The model under review builds one solid part; all positions refer to its coordinate system, in mm. A direction names the side the tool comes from. Give positions to 0.01 mm unless a question says otherwise; leave off trailing zeros. Order: outer loops, then holes, each group sorted by start corner. A loop starts at its lowest first (then second) coordinate and runs counter-clockwise, first axis right, second up.
```python
from build123d import *

# Parameters (mm, degrees)
SKETCH1_W           = 160
SKETCH1_H           = 104
SKETCH1_R           = 2.5
BOSS_EXTRUDE1_DEPTH = 28.45
CUT_EXTRUDE1_DEPTH  = 135.258714801
SKETCH5_W           = 60
SKETCH5_H           = 104
BOSS_EXTRUDE2_DEPTH = 5
SKETCH3_R           = 4.8
CUT_EXTRUDE2_DEPTH  = 7
CUT_EXTRUDE3_START  = 6.5
SKETCH4_R           = 4.8
CUT_EXTRUDE3_DEPTH  = 13.35
SKETCH6_R           = 2.5
CUT_EXTRUDE4_DEPTH  = 100.566071028
SKETCH7_R           = 2.1
CUT_EXTRUDE5_DEPTH  = 12
CUT_EXTRUDE6_START  = -12
SKETCH8_R           = 2.1
CUT_EXTRUDE6_DEPTH  = 12
SKETCH9_R           = 3.75
CUT_EXTRUDE7_DEPTH  = 26


with BuildPart() as part:
    # Sketch1 → Boss-Extrude1 (new body)
    with BuildSketch(Plane.XY):
        Rectangle(SKETCH1_W, SKETCH1_H)
        with Locations((20, -37)):
            Circle(SKETCH1_R, mode=Mode.SUBTRACT)
        with Locations(Location((-20, -37, 0), (0, 0, 180))):
            Circle(SKETCH1_R, mode=Mode.SUBTRACT)
        with Locations((20, -17)):
            Circle(SKETCH1_R, mode=Mode.SUBTRACT)
        with Locations((20, 3)):
            Circle(SKETCH1_R, mode=Mode.SUBTRACT)
        with Locations(Location((-20, 3, 0), (0, 0, 180))):
            Circle(SKETCH1_R, mode=Mode.SUBTRACT)
        with Locations(Location((-20, -17, 0), (0, 0, 180))):
            Circle(SKETCH1_R, mode=Mode.SUBTRACT)
    extrude(amount=BOSS_EXTRUDE1_DEPTH)

    # Sketch2 → Cut-Extrude1 (cut, through all)
    with BuildSketch(Plane(origin=(0, 52, 0), x_dir=(1, 0, 0), z_dir=(0, 1, 0))):
        Polygon((-3.95, -28.45), (3.95, -28.45), (3.95, -21.95), (7, -21.95), (7, -15.45), (-7, -15.45), (-7, -21.95), (-3.95, -21.95), align=None)
        Polygon((25.85, -28.45), (25.85, -21.95), (28.9, -21.95), (28.9, -15.45), (14.9, -15.45), (14.9, -21.95), (17.95, -21.95), (17.95, -28.45), align=None)
        Polygon((47.75, -28.45), (47.75, -21.95), (50.8, -21.95), (50.8, -15.45), (36.8, -15.45), (36.8, -21.95), (39.85, -21.95), (39.85, -28.45), align=None)
        Polygon((69.65, -28.45), (69.65, -21.95), (72.7, -21.95), (72.7, -15.45), (58.7, -15.45), (58.7, -21.95), (61.75, -21.95), (61.75, -28.45), align=None)
        Polygon((-28.9, -15.45), (-28.9, -21.95), (-25.85, -21.95), (-25.85, -28.45), (-17.95, -28.45), (-17.95, -21.95), (-14.9, -21.95), (-14.9, -15.45), align=None)
        Polygon((-50.8, -15.45), (-50.8, -21.95), (-47.75, -21.95), (-47.75, -28.45), (-39.85, -28.45), (-39.85, -21.95), (-36.8, -21.95), (-36.8, -15.45), align=None)
        Polygon((-72.7, -15.45), (-72.7, -21.95), (-69.65, -21.95), (-69.65, -28.45), (-61.75, -28.45), (-61.75, -21.95), (-58.7, -21.95), (-58.7, -15.45), align=None)
    extrude(amount=-CUT_EXTRUDE1_DEPTH, mode=Mode.SUBTRACT)

    # Sketch5 → Boss-Extrude2 (add)
    with BuildSketch(Plane(origin=(0, 0, 0), x_dir=(-1, 0, 0), z_dir=(0, 0, -1))):
        Rectangle(SKETCH5_W, SKETCH5_H)
    extrude(amount=BOSS_EXTRUDE2_DEPTH)

    # Sketch3 → Cut-Extrude2 (cut)
    with BuildSketch(Plane.XY.offset(28.45)):
        with Locations((-20, 3)):
            Circle(SKETCH3_R)
        with Locations((20, 3)):
            Circle(SKETCH3_R)
        with Locations((-20, -17)):
            Circle(SKETCH3_R)
        with Locations((20, -17)):
            Circle(SKETCH3_R)
        with Locations((-20, -37)):
            Circle(SKETCH3_R)
        with Locations((20, -37)):
            Circle(SKETCH3_R)
    extrude(amount=-CUT_EXTRUDE2_DEPTH, mode=Mode.SUBTRACT)

    # Sketch4 → Cut-Extrude3 (cut)
    with BuildSketch(Plane.XY.offset(15.45).offset(CUT_EXTRUDE3_START)):
        with Locations((-20, 3)):
            Circle(SKETCH4_R)
        with Locations((20, 3)):
            Circle(SKETCH4_R)
        with Locations((-20, -17)):
            Circle(SKETCH4_R)
        with Locations((20, -17)):
            Circle(SKETCH4_R)
        with Locations((-20, -37)):
            Circle(SKETCH4_R)
        with Locations((20, -37)):
            Circle(SKETCH4_R)
    extrude(amount=-CUT_EXTRUDE3_DEPTH, mode=Mode.SUBTRACT)

    # Sketch6 → Cut-Extrude4 (cut, through all)
    with BuildSketch(Plane.XY):
        with Locations((-20, 3)):
            Circle(SKETCH6_R)
        with Locations((20, 3)):
            Circle(SKETCH6_R)
        with Locations((-20, -17)):
            Circle(SKETCH6_R)
        with Locations((20, -17)):
            Circle(SKETCH6_R)
        with Locations((20, -37)):
            Circle(SKETCH6_R)
        with Locations((-20, -37)):
            Circle(SKETCH6_R)
    extrude(amount=-CUT_EXTRUDE4_DEPTH, mode=Mode.SUBTRACT)

    # Sketch7 → Cut-Extrude5 (cut)
    with BuildSketch(Plane(origin=(0, 52, 0), x_dir=(1, 0, 0), z_dir=(0, 1, 0))):
        with Locations(Location((-70, -8, 0), (0, 0, 180))):
            Circle(SKETCH7_R)
        with Locations(Location((-30, -8, 0), (0, 0, 180))):
            Circle(SKETCH7_R)
        with Locations((70, -8)):
            Circle(SKETCH7_R)
        with Locations((30, -8)):
            Circle(SKETCH7_R)
    extrude(amount=-CUT_EXTRUDE5_DEPTH, mode=Mode.SUBTRACT)

    # Sketch8 → Cut-Extrude6 (cut)
    with BuildSketch(Plane.XZ.offset(52).offset(CUT_EXTRUDE6_START)):
        with Locations((70, 8)):
            Circle(SKETCH8_R)
        with Locations((30, 8)):
            Circle(SKETCH8_R)
        with Locations(Location((-30, 8, 0), (0, 0, 180))):
            Circle(SKETCH8_R)
        with Locations(Location((-70, 8, 0), (0, 0, 180))):
            Circle(SKETCH8_R)
    extrude(amount=CUT_EXTRUDE6_DEPTH, mode=Mode.SUBTRACT)

    # Sketch9 → Cut-Extrude7 (cut)
    with BuildSketch(Plane.XY.offset(28.45)):
        with Locations((-65, 11)):
            Circle(SKETCH9_R)
        with Locations((-65, -37)):
            Circle(SKETCH9_R)
        with Locations((65, -37)):
            Circle(SKETCH9_R)
        with Locations((65, 11)):
            Circle(SKETCH9_R)
    extrude(amount=-CUT_EXTRUDE7_DEPTH, mode=Mode.SUBTRACT)


solid = part.part
```
1. For faces 1 (the flat face through (66, 1, 15.45)), 2 (the cylindrical face through (71.13, 46.08, 6.23)), 3 (the cylindrical face through (-15.2, -37.1, 25.2)), list the 3-axis set-ups (+Z, -Z, +X, -X, +Y, -Y) from which the entire face can be reached by the end or side of a thin tool; tool diameter is ignored.
2. Take a section at B-B (x = 65). Write out the cut boundary in (y, z).
3. To check wall thickness, follow line 1 (X direction, y = -17, z = 5.25); line 2 (Y direction, x = -20, z = 12); line 3 (X direction, y = -37, z = -3.35). State the ranges of each line that lie inside material, in increasing order.
4. Insertion check: pin 1 (4.5 mm diameter, centred on x = 20, y = -17, fed in from -Z); pin 2 (2.5 mm diameter, centred on y = -22, z = -1.5, fed in from -X); pin 3 (2 mm diameter, centred on x = 46, y = -28, fed in from -Z); pin 4 (4 mm diameter, centred on x = -65, y = 10.5, fed in from +Z). Each pin has a flat end and moves straight along its axis. Give the tip position at first contact, or say it passes through.
5. Draft analysis for pull direction Z (two halves, no side actions). For faces 4 (the flat face through (-75, 1, 28.45)), 5 (the flat face through (38, 1, 21.95)), 6 (the cylindrical face through (16.19, 0.08, 12.07)), state which applies: pulls with the +Z half, pulls with the -Z half, needs draft (parallel to the pull), parting line crosses it, or undercut.
6. Take a section at A-A (x = -20). Write out the cut boundary in (y, z).
7. Take a section at C-C (z = 25.5). Count the separate pieces of the cut face and the enclosed holes in it, and give its area (3 significant figures).
Answer:
1. face 1: +Y, -Y
1. face 2: +Y
1. face 3: +Z
2. outline: (-52, 0) - (52, 0) - (52, 15.45) - (14.75, 15.45) - (14.75, 2.45) - (7.25, 2.45) - (7.25, 15.45) - (-33.25, 15.45) - (-33.25, 2.45) - (-40.75, 2.45) - (-40.75, 15.45) - (-52, 15.45) - close
3. line 1: x = -80 to -22.5, -17.5 to 17.5, 22.5 to 80
3. line 2: y = -52 to -41.8, -32.2 to -21.8, -12.2 to -1.8, 7.8 to 52
3. line 3: x = -30 to -22.5, -17.5 to 17.5, 22.5 to 30
4. pin 1: passes through
4. pin 2: stops at x = -30
4. pin 3: stops at z = 0
4. pin 4: stops at z = 2.45
5. face 4: pulls with the +Z half
5. face 5: undercut
5. face 6: needs draft
6. outline: (-52, -5) - (-39.5, -5) - (-39.5, 8.6) - (-41.8, 8.6) - (-41.8, 15.45) - (-52, 15.45) - close; (-34.5, -5) - (-19.5, -5) - (-19.5, 8.6) - (-21.8, 8.6) - (-21.8, 15.45) - (-32.2, 15.45) - (-32.2, 8.6) - (-34.5, 8.6) - close; (-14.5, -5) - (0.5, -5) - (0.5, 8.6) - (-1.8, 8.6) - (-1.8, 15.45) - (-12.2, 15.45) - (-12.2, 8.6) - (-14.5, 8.6) - close; (5.5, -5) - (52, -5) - (52, 15.45) - (7.8, 15.45) - (7.8, 8.6) - (5.5, 8.6) - close
7. separate pieces: 8
7. enclosed holes: 0
7. area: 10,800 mm2
